```python
from build123d import *

# Parameters (mm, degrees)
SKETCH002_R   = 4.252865
SKETCH002_R_2 = 5.59623
SKETCH002_R_3 = 4.877243
SKETCH002_R_4 = 5.047412
PAD001_DEPTH  = 20
PAD_DEPTH     = 80
SKETCH001_W   = 100
SKETCH001_H   = 80
POCKET_DEPTH  = 14.001


with BuildPart() as pad001:
    # Sketch002 → Pad001 (new body)
    with BuildSketch(Plane.XZ):
        with Locations((-31.93054, 65.612114)):
            Circle(SKETCH002_R)
        with Locations((-9.299617, 59.023361)):
            Circle(SKETCH002_R_2)
        with Locations((4.772683, 62.008789)):
            Circle(SKETCH002_R_3)
        with Locations((23.342754, 60.151779)):
            Circle(SKETCH002_R_4)
    extrude(amount=-PAD001_DEPTH)


with BuildPart() as cut:
    # Sketch → Pad (new body)
    with BuildSketch(Plane.XY):
        with BuildLine():
            Line((45, 0), (50, 0))
            ThreePointArc((50, 0), (0, 14), (-50, 0))
            Line((-50, 0), (-45, 0))
            ThreePointArc((-45, 0), (0, 10.917116), (45, 0))
        make_face()
    extrude(amount=PAD_DEPTH)

    # Sketch001 → Pocket (cut, through all)
    with BuildSketch(Plane.XZ):
        with Locations((0, 40)):
            Rectangle(SKETCH001_W, SKETCH001_H)
        Polygon((-30.718987, 4.784545), (-48.360384, 16.897081), (-48.360384, 76.077912), (45.416021, 76.077912), (45.416021, 15.337389), (35.539104, 4.784545), align=None, mode=Mode.SUBTRACT)
    extrude(amount=-POCKET_DEPTH, mode=Mode.SUBTRACT)

    # Cut: cut Pad001
    add(pad001.part, mode=Mode.SUBTRACT)


solid = cut.part
```
Can you work these out from the model? Positions are in its coordinate system, mm. Round coordinates to 2 decimals unless told otherwise and drop trailing zeros. Order: outer loops, then holes, each group sorted by start corner. A loop starts at its lowest first (then second) coordinate and runs counter-clockwise, first axis right, second up. Notation, with made-up numbers: (-6.75, 22.25) -> (2.25, 22.25) arc R17 ccw to (2.25, 43.25) -> close; hole circle Ø1 at (-4.75, -20.5). An arc over 180 degrees is marked (long way). Return JSON: item names as keys, results as strings. Group by question number.
1. I need wall thicknesses on line 1 (X direction, y = 3.25, z = 27); line 2 (Y direction, x = 2, z = 52.5); line 3 (Z direction, x = 28, y = 9). Which ranges of each line are inside material? Lowest first, please. Write a range as [from, to].
2. Will these pins go through, and if not, where does the flat tip stop? pin 1 (4 mm diameter, centred on y = 5, z = 18.5, fed in from +X); pin 2 (5 mm diameter, centred on x = 10.5, z = 45, fed in from +Y); pin 3 (1 mm diameter, centred on y = 12, z = 56, fed in from +X).
3. If we section it at A-A, the plane z = 21: Write out the boundary of the cut face in (x, y), then the cut area to 3 significant figures.
4. We'd pull the mould along X, two halves only. Please class faces 1 (the face through (-0.654, 10.915, 39.932)), 2 (the face through (40.547, 3.55, 10.135)), 3 (the face through (-4.13, 11.83, 56.88)), 4 (the face through (-1, 13.995, 39.932)): released by +X, released by -X, zero draft, split by the parting line, or undercut.
5. If we section it at B-B, the plane z = 13.5: Write out the boundary of the cut face in (x, y), then the cut area to 3 significant figures.
Output values:
{
 "1": {"line 1": "[-44.21, -38.04], [38.04, 44.21]", "line 2": "[10.9, 13.98]", "line 3": "[4.78, 58.21], [62.1, 76.08]"},
 "2": {"pin 1": "x = 44.69", "pin 2": "y = 13.67", "pin 3": "x = 21.09"},
 "3": {"outline": "(-48.36, 0) -> (-45, 0) arc R98.2 cw to (45, 0) -> (45.42, 0) -> (45.42, 2.62) arc R96.29 ccw to (-48.36, 0.97) -> close", "area": "278 mm²"},
 "4": {"face 1": "undercut", "face 2": "released by +X", "face 3": "undercut", "face 4": "split by the parting line"},
 "5": {"outline": "(-43.41, 0.8) arc R98.2 cw to (43.7, 0.66) -> (43.7, 3.51) arc R96.29 ccw to (-43.41, 3.66) -> close", "area": "262 mm²"}
}
